Autodesk Inventor part; units mm, degrees
ref_plane "YZ Plane" through (0, 0, 0) normal (1, 0, 0) x (0, 1, 0)
ref_plane "XZ Plane" through (0, 0, 0) normal (0, 1, 0) x (-1, 0, 0)
ref_plane "XY Plane" through (0, 0, 0) normal (0, 0, 1) x (1, 0, 0)
sketch "스케치1" plane through (0, 0, 0) normal (0, 1, 0) x (-1, 0, 0)
  line L0 (23, -56) -> (-23, -56)
  line L1 (-23, -56) -> (-23, 56)
  line L2 (-23, 56) -> (23, 56)
  line L3 (23, 56) -> (23, -56)
  point P0 (0, 0)
  dimension "d0" = 112
  dimension "d1" = 56
  dimension "d2" = 46
  dimension "d3" = 23
extrude "돌출1" add sketch "스케치1" along normal blind 16.1
sketch "스케치2" plane through (0, 0, 0) normal (0, -1, 0) x (1, 0, 0)
  circle A0 centre (0, 0) radius 14.52
  dimension "d6" = 29.04
extrude "돌출2" cut sketch "스케치2" against normal blind 0.5
sketch "스케치3" plane through (0, 0.5, 0) normal (0, -1, 0) x (1, 0, 0)
  circle A0 centre (0, 0) radius 5.075
  circle A1 centre (0, 11) radius 1.25
  circle A2 centre (-7.7782, 7.7782) radius 1.25
  circle A3 centre (-11, 0) radius 1.25
  circle A4 centre (-7.7782, -7.7782) radius 1.25
  circle A5 centre (0, -11) radius 1.25
  circle A6 centre (7.7782, -7.7782) radius 1.25
  circle A7 centre (11, 0) radius 1.25
  circle A8 centre (7.7782, 7.7782) radius 1.25
  dimension "d9" = 10.15
  dimension "d10" = 2.5
  dimension "d11" = 11
  dimension "d14" = 360
extrude "돌출3" cut sketch "스케치3" against normal blind 30
sketch "스케치4" plane through (0, 16.1, 0) normal (0, 1, 0) x (1, 0, 0)
  circle A0 centre (0, -11) radius 1.25
  circle A1 centre (0, -11) radius 3
  circle A2 centre (7.7782, -7.7782) radius 3
  circle A3 centre (11, 0) radius 3
  circle A4 centre (7.7782, 7.7782) radius 3
  circle A5 centre (0, 11) radius 3
  circle A6 centre (-7.7782, 7.7782) radius 3
  circle A7 centre (-11, 0) radius 3
  circle A8 centre (-7.7782, -7.7782) radius 3
  point P0 (0, 0)
  dimension "d18" = 6
  dimension "d21" = 360
extrude "돌출4" cut sketch "스케치4" against normal blind 5 contours A0 | A1 | A2 | A3 | A4 | A5 | A6 | A7 | A8
sketch "스케치5" plane through (0, 16.1, 0) normal (0, 1, 0) x (1, 0, 0)
  line L0 (-23, -56) -> (23, -56)
  line L1 (23, -56) -> (23, -51)
  line L2 (23, -51) -> (-23, -51)
  line L3 (-23, -51) -> (-23, -56)
  line L4 (-23, -56) -> (23, -56)
  line L5 (-14.52, -51) -> (14.52, -51)
  line L6 (14.52, -51) -> (14.52, -56)
  line L7 (14.52, -56) -> (-14.52, -56)
  line L8 (-14.52, -56) -> (-14.52, -51)
  line L9 (0, 0) -> (-19.344, 0)
  line L10 (-23, 56) -> (23, 56)
  line L11 (23, 56) -> (23, 51)
  line L12 (23, 51) -> (-23, 51)
  line L13 (-23, 51) -> (-23, 56)
  line L14 (-23, 56) -> (23, 56)
  line L15 (-14.52, 51) -> (14.52, 51)
  line L16 (14.52, 51) -> (14.52, 56)
  line L17 (14.52, 56) -> (-14.52, 56)
  line L18 (-14.52, 56) -> (-14.52, 51)
  point P0 (-23, 56)
  dimension "d25" = 5
  dimension "d27" = 29.04
  dimension "d28" = 14.52
extrude "돌출5" add sketch "스케치5" along normal blind 61.1 contours L3 L2 L8 L0 | L6 L2 L1 L0 | L10 L18 L12 L13 | L10 L11 L12 L16
sketch "스케치6" plane through (0, 16.1, 0) normal (0, 1, 0) x (1, 0, 0)
  line L0 (-23, -56) -> (-23, 56)
  line L1 (-23, -16.98) -> (-14.52, -16.98)
  line L2 (-14.52, 16.98) -> (-23, 16.98)
  line L3 (-14.52, -51) -> (-23, -51)
  line L4 (-23, 51) -> (-14.52, 51)
  line L5 (-23, -16.98) -> (-14.52, -16.98)
  line L6 (-14.52, -16.98) -> (-14.52, -11.98)
  line L7 (-14.52, -11.98) -> (-23, -11.98)
  line L8 (-23, -11.98) -> (-23, -16.98)
  line L9 (-23, 16.98) -> (-14.52, 16.98)
  line L10 (-14.52, 16.98) -> (-14.52, 11.98)
  line L11 (-14.52, 11.98) -> (-23, 11.98)
  line L12 (-23, 11.98) -> (-23, 16.98)
  circle A0 centre (0, 0) radius 14.52
  line L13 (0, 0) -> (0, -35.0493)
  line L14 (23, -16.98) -> (14.52, -16.98)
  line L15 (14.52, 16.98) -> (23, 16.98)
  line L16 (23, -16.98) -> (14.52, -16.98)
  line L17 (14.52, -16.98) -> (14.52, -11.98)
  line L18 (14.52, -11.98) -> (23, -11.98)
  line L19 (23, -11.98) -> (23, -16.98)
  line L20 (23, 16.98) -> (14.52, 16.98)
  line L21 (14.52, 16.98) -> (14.52, 11.98)
  line L22 (14.52, 11.98) -> (23, 11.98)
  line L23 (23, 11.98) -> (23, 16.98)
  dimension "d31" = 34.02
  dimension "d32" = 34.02
  dimension "d34" = 5
  dimension "d35" = 5
  dimension "d36" = 8.48
  dimension "d37" = 8.48
extrude "돌출6" add sketch "스케치6" along normal blind 61.1 contours L0 L2 L10 L11 | L0 L7 L6 L1 | L14 L17 L18 L19 | L15 L23 L22 L21
sketch "스케치7" plane through (0, 16.1, 0) normal (0, 1, 0) x (1, 0, 0)
  line L0 (-14.52, -51) -> (-14.52, -56)
  line L1 (14.52, -51) -> (23, -51)
  line L2 (-14.52, -56) -> (14.52, -56)
  line L3 (14.52, -56) -> (14.52, -51)
  line L4 (14.52, -51) -> (-14.52, -51)
  line L5 (-14.52, -51) -> (-14.52, -56)
  line L6 (-14.52, 51) -> (-23, 51)
  line L7 (14.52, 51) -> (14.52, 56)
  line L8 (-14.52, 51) -> (14.52, 51)
  line L9 (14.52, 51) -> (14.52, 56)
  line L10 (14.52, 56) -> (-14.52, 56)
  line L11 (-14.52, 56) -> (-14.52, 51)
  line L12 (-23, -16.98) -> (-23, -51)
  line L13 (-23, -16.98) -> (-14.52, -16.98)
  line L14 (-23, -51) -> (-20, -51)
  line L15 (-20, -51) -> (-20, -16.98)
  line L16 (-20, -16.98) -> (-23, -16.98)
  line L17 (-23, -16.98) -> (-23, -51)
  line L18 (-23, 16.98) -> (-14.52, 16.98)
  line L19 (-23, 16.98) -> (-20, 16.98)
  line L20 (-20, 16.98) -> (-20, 51)
  line L21 (-20, 51) -> (-23, 51)
  line L22 (-23, 51) -> (-23, 16.98)
  line L23 (23, 56) -> (23, -56)
  line L24 (23, 51) -> (20, 51)
  line L25 (20, 51) -> (20, 16.98)
  line L26 (20, 16.98) -> (23, 16.98)
  line L27 (23, 16.98) -> (23, 51)
  line L28 (23, -51) -> (23, -16.98)
  line L29 (23, -16.98) -> (20, -16.98)
  line L30 (20, -16.98) -> (20, -51)
  line L31 (20, -51) -> (23, -51)
  line L32 (23, -51) -> (23, -16.98)
  point P0 (0, 0)
  dimension "d40" = 3
  dimension "d41" = 3
  dimension "d42" = 3
  dimension "d43" = 3
extrude "돌출7" add sketch "스케치7" along normal blind 5.6
sketch "스케치8" plane through (0, 16.1, 0) normal (0, 1, 0) x (1, 0, 0)
  line L0 (23, 11.98) -> (14.52, 11.98)
  line L1 (23, -11.98) -> (14.52, -11.98)
  line L2 (14.52, -11.98) -> (14.52, 11.98)
  line L3 (14.52, 11.98) -> (23, 11.98)
  line L4 (23, 11.98) -> (23, -11.98)
  line L5 (-23, 11.98) -> (-23, -11.98)
  line L6 (-14.52, -11.98) -> (-14.52, -16.98)
  line L7 (-23, 11.98) -> (-14.52, 11.98)
  line L8 (-14.52, 11.98) -> (-14.52, -11.98)
  line L9 (-14.52, -11.98) -> (-23, -11.98)
  line L10 (-23, -11.98) -> (-23, 11.98)
  point P0 (0, 0)
extrude "돌출8" add sketch "스케치8" along normal blind 25
sketch "스케치9" plane through (-23, 0, 56) normal (0, 0, 1) x (1, 0, 0)
  circle A0 centre (5.8, 68.2) radius 1.35
  line L0 (0, 77.2) -> (8.48, 77.2)
  line L1 (0, 0) -> (0, 77.2)
  circle A1 centre (5.8, 46.2) radius 1.35
  line L2 (23, 0) -> (23, 16.9494)
  circle A2 centre (40.2, 68.2) radius 1.35
  circle A3 centre (40.2, 46.2) radius 1.35
  dimension "d48" = 9
  dimension "d49" = 5.8
  dimension "d50" = 22
  dimension "d51" = 2.7
  dimension "d52" = 2.7
  dimension "d53" = 5.8
extrude "돌출9" cut sketch "스케치9" against normal blind 300
equation "\"TransitionRadius\" = BendRadius"
properties part number "shoulder_5"
The listing builds one solid part. Answer for the finished solid, in the listing's coordinates (mm). A direction names the side the tool comes from. Coordinates: 2 decimals unless noted, no trailing zeros. Loops run counter-clockwise (first coordinate to the right, second up) from the corner with the lowest first, then second, coordinate; pieces in that order, holes last. Notation, with made-up numbers: (-37, 38) -> (-12, 38) arc R16 ccw to (-12, 66) -> close; hole circle Ø3 at (-24, 22). An arc over 180 degrees is marked (long way). Use one line per item in the form item = value. Start each with the question number.
Item 1: The mould has two halves that part along Z. Classify faces 6 (the face through (6, 0.5, 0)), 7 (the face through (-19, 77.2, 14)): released by +Z, released by -Z, zero draft, split by the parting line, or undercut.
Item 2: Flat-ended cylindrical pins translate along their axes: pin 1 Ø1.5 at (x, z) = (-14, 38) entering from +Y; pin 2 Ø3.5 at (x, z) = (7.78, 7.78) entering from -Y; pin 3 Ø1.8 at (x, z) = (-11, -1.5) entering from +Y. Find the tip coordinate at first contact, or state that the pin passes through.
Item 3: The part is cut by section B-B on x = 0. Count the separate pieces of the cut face and the enclosed holes in it, then the cut area to 3 significant figures.
Item 4: Consider L1, parallel to X at y = 68.2, z = 54.8; L2, parallel to Z at x = 20.5, y = 31; L3, parallel to Y at x = -17.2, z = 15.3. Determine where each line is inside the solid, lowest interval first. Write a range as [from, to].
Item 5: A tool of negligible diameter and unlimited length cuts with its end or side. For faces 1 (the face through (0, 21.7, -54)), 2 (the face through (19, 59, 11.98)), 3 (the face through (5.57, 13.64, 5.75)), 4 (the face through (-19, 77.2, -15)), 5 (the face through (17.82, 67, -53.46)), from which of +Z, -Z, +X, -X, +Y, -Y can it reach the whole face along a straight path? Write none if from no direction.
Item 6: The part is cut by section A-A on y = 27.5. Determine the outline of the cut face in (x, z), then the cut area to 3 significant figures.
Answer key:
q1.face_6 = undercut
q1.face_7 = zero draft
q2.pin_1 = 16.1
q2.pin_2 = 0.5
q2.pin_3 = 11.1
q3.separate_pieces = 4
q3.enclosed_holes = 0
q3.area = 1,570 mm2
q4.L1 = [-23, -18.55], [-15.85, -14.52], [14.52, 15.85], [18.55, 23]
q4.L2 = [-56, -51], [-16.98, 16.98], [51, 56]
q4.L3 = [0, 44.85], [47.55, 66.85], [69.55, 77.2]
q5.face_1 = +Z, -Z, +Y
q5.face_2 = +X, -X, +Y
q5.face_3 = +Y
q5.face_4 = +Z, -Z, +X, -X, +Y
q5.face_5 = +Z, -Z
q6.outline = (-23, -56) -> (-14.52, -56) -> (-14.52, -51) -> (-23, -51) -> close; (-23, -16.98) -> (-14.52, -16.98) -> (-14.52, 16.98) -> (-23, 16.98) -> close; (-23, 51) -> (-14.52, 51) -> (-14.52, 56) -> (-23, 56) -> close; (14.52, -56) -> (23, -56) -> (23, -51) -> (14.52, -51) -> close; (14.52, -16.98) -> (23, -16.98) -> (23, 16.98) -> (14.52, 16.98) -> close; (14.52, 51) -> (23, 51) -> (23, 56) -> (14.52, 56) -> close
q6.area = 746 mm2
